The model under review builds one solid part; all positions refer to its coordinate system, in mm. A direction names the side the tool comes from. Coordinates: 2 decimals unless noted, no trailing zeros. Order: outer loops, then holes, each group sorted by start corner. A loop starts at its lowest first (then second) coordinate and runs counter-clockwise, first axis right, second up. Notation, with made-up numbers: M 62,24 L 111,24 A15 cw 111,50 Z; hole C 89.5,-4 d1. An arc over 180 degrees is marked long. Write each question's results on one line, items separated by ' | '.
from build123d import *
from build123d.topology import SkipClean

# Parameters (mm, degrees)
SKETCH1_R           = 19.25
SKETCH1_R_2         = 17.75
BOSS_EXTRUDE1_DEPTH = 25
BOSS_EXTRUDE2_START = 1
SKETCH2_R           = 19.25
BOSS_EXTRUDE2_DEPTH = 1
CUT_EXTRUDE1_DEPTH  = 38.644720745
FILLET2_R           = 1.5


with BuildPart() as part:
    # Sketch1 → Boss-Extrude1 (new body)
    with BuildSketch(Plane.XY):
        Circle(SKETCH1_R)
        Circle(SKETCH1_R_2, mode=Mode.SUBTRACT)
    extrude(amount=BOSS_EXTRUDE1_DEPTH)

    # Sketch2 → Boss-Extrude2 (add)
    with BuildSketch(Plane(origin=(0, 0, 0), x_dir=(-1, 0, 0), z_dir=(0, 0, -1)).offset(BOSS_EXTRUDE2_START)):
        Circle(SKETCH2_R)
    extrude(amount=-BOSS_EXTRUDE2_DEPTH)

    # Sketch3 → Cut-Extrude1 (cut, through all)
    with SkipClean():  # the faces are left unmerged after this step: merging them gives an invalid solid
        with BuildSketch(Plane(origin=(0, 0, -1), x_dir=(-1, 0, 0), z_dir=(0, 0, -1))):
            with BuildLine():
                Line((-16.235285332, 10.343017461), (0, 0))
                Line((0, 0), (16.235285332, 10.343017461))
                ThreePointArc((16.235285332, 10.343017461), (0, 19.25), (-16.235285332, 10.343017461))
            make_face()
        extrude(amount=-CUT_EXTRUDE1_DEPTH, mode=Mode.SUBTRACT)

    # Fillet2
    fillet2_edges = [part.edges().sort_by_distance(p)[0] for p in [
        (-4.966964999, -17.040884915, 0),
    ]]
    fillet(fillet2_edges, radius=FILLET2_R)


solid = part.part
1) Take a section at A-A on z = 3. State the section outline as (x, y) points.
Solutions:
outline: M -16.24,10.34 A19.25 ccw long 16.24,10.34 L 14.97,9.54 A17.75 cw long -14.97,9.54 Z
2) For faces 1 (the flat face through (-15.295, 9.744, 8.087)), 2 (the cylindrical face through (-0.531, -17.742, 13.086)), 3 (the flat face through (3, -18, 25)), list the 3-axis set-ups (+Z, -Z, +X, -X, +Y, -Y) from which the entire face can be reached by the end or side of a thin tool; tool diameter is ignored.
Solutions:
face 1: +Z, -Z, +Y | face 2: +Z | face 3: +Z, +X, -X, +Y, -Y
3) For pin 1 (3 mm diameter, centred on x = -12, z = 22, fed in from +Y); pin 2 (5 mm diameter, centred on y = -9, z = 5, fed in from +X); pin 3 (12 mm diameter, centred on x = -11.5, y = -12, fed in from +Z); pin 4 (10 mm diameter, centred on x = -6.5, y = 0.5, fed in from +Z), all flat-tipped, find the tip position at first contact; note any pin that passes through.
Solutions:
pin 1: y = -11.52 | pin 2: x = 18.12 | pin 3: z = 25 | pin 4: z = 0
4) The part is to be moulded in two halves that separate along X. For faces 4 (the flat face through (0, -4, -1)), 5 (the flat face through (0, -4, 0)), say which applies: pulls with the +X half, pulls with the -X half, needs draft (parallel to the pull), parting line crosses it, or undercut.
Solutions:
face 4: needs draft | face 5: undercut
5) To check wall thickness, follow line 1 along X through (y, z) = (0, 12.25); line 2 along Y through (x, z) = (-16, 10); line 3 along Z through (x, y) = (3.5, -4). State the ranges of each line that lie inside material, in increasing order.
Solutions:
line 1: -19.25 to -17.75, 17.75 to 19.25 | line 2: -10.7 to -7.69, 7.69 to 10.19 | line 3: -1 to 0
